from build123d import *

# Parameters (mm, degrees)
SKETCH1_R           = 47.5
BOSS_EXTRUDE1_DEPTH = 200
SKETCH2_R           = 30
CUT_EXTRUDE2_DEPTH  = 200
SKETCH4_R           = 47.5
BOSS_EXTRUDE2_DEPTH = 62.5
SKETCH5_R           = 5
CUT_EXTRUDE3_DEPTH  = 20
SKETCH6_R           = 27
CUT_EXTRUDE4_DEPTH  = 4


with BuildPart() as part:
    # Sketch1 → Boss-Extrude1 (new body)
    with BuildSketch(Plane(origin=(0, 0, 0), x_dir=(1, 0, 0), z_dir=(0, 1, 0))):
        with Locations(Location((0, 0, 0), (0, 0, 270))):
            Circle(SKETCH1_R)
    extrude(amount=BOSS_EXTRUDE1_DEPTH)

    # Sketch2 → Cut-Extrude2 (cut)
    with BuildSketch(Plane(origin=(0, 200, 0), x_dir=(1, 0, 0), z_dir=(0, 1, 0))):
        with Locations(Location((0, 0, 0), (0, 0, 270))):
            Circle(SKETCH2_R)
    extrude(amount=-CUT_EXTRUDE2_DEPTH, mode=Mode.SUBTRACT)

    # Sketch4 → Boss-Extrude2 (add)
    with BuildSketch(Plane.XY):
        with Locations((0, 100)):
            Circle(SKETCH4_R)
    extrude(amount=BOSS_EXTRUDE2_DEPTH)

    # Sketch5 → Cut-Extrude3 (cut)
    with BuildSketch(Plane.XY.offset(62.5)):
        with Locations((0, 138)):
            Circle(SKETCH5_R)
        with Locations((0, 62)):
            Circle(SKETCH5_R)
        with Locations((38, 100)):
            Circle(SKETCH5_R)
        with Locations((-38, 100)):
            Circle(SKETCH5_R)
    extrude(amount=-CUT_EXTRUDE3_DEPTH, mode=Mode.SUBTRACT)

    # Sketch6 → Cut-Extrude4 (cut)
    with BuildSketch(Plane.XY.offset(62.5)):
        with Locations((0, 100)):
            Circle(SKETCH6_R)
    extrude(amount=-CUT_EXTRUDE4_DEPTH, mode=Mode.SUBTRACT)


solid = part.part
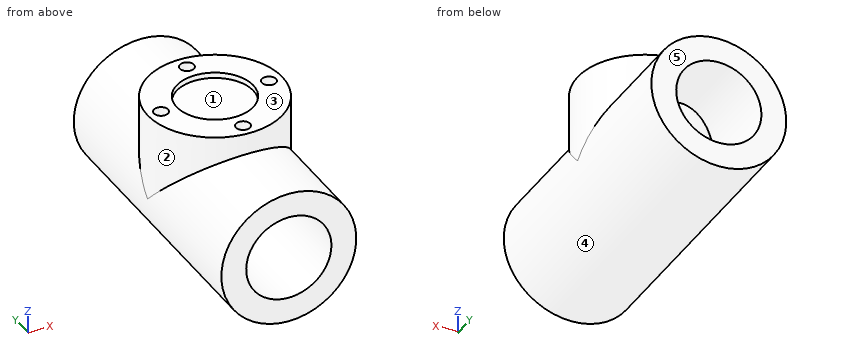
Source: CAD feature listing. Evaluate the final solid. Frame: model axes, mm. Face numbers are marked on the shaded views. A direction names the side the tool comes from. Give positions to 0.01 mm unless a question says otherwise; leave off trailing zeros. Loops run counter-clockwise (first coordinate to the right, second up) from the corner with the lowest first, then second, coordinate; pieces in that order, holes last. Notation, with made-up numbers: (51.25, 63.5) -> (74.25, 63.5) arc R22 ccw to (74.25, 82.5) -> close; hole circle Ø5 at (46, -30). An arc over 180 degrees is marked (long way). Use a Markdown table: item, result. Add a question column.
1) Reachability of the marked faces 4 and 5 from +Z, -Z, +X, -X, +Y, -Y: full face, straight path, thin tool, end or side. Return the list, or none.
2) First-contact query: pin 1 (12 mm diameter, centred on y = 60.5, z = -21, fed in from +X); pin 2 (5 mm diameter, centred on x = -37, y = 102, fed in from +Z); pin 3 (5 mm diameter, centred on y = 44.5, z = 45, fed in from -X). Flat tips, straight axial feed; report the tip coordinate or a pass-through.
3) Section query C-C, the plane x = -38. Return the cut outline in (y, z), then the cut area to 3 significant figures.
4) Pull-direction query (X, two-part tool) for the marked faces 1, 2 and 3; classes: +X half, -X half, draft (parallel to the pull), parting line (faces both ways), or undercut.
5) Section query D-D, the plane z = -23.5. Return the cut outline in (x, y), then the cut area to 3 significant figures.
6) Section query A-A, the plane x = 0. Return the cut outline in (y, z).
7) Line query: line 1 along Y through (x, z) = (0, 59); line 2 along Z through (x, y) = (-12, 88.5); line 3 along Z through (x, y) = (27.5, 104). Output: solid intervals per line, ascending. Write a range as [from, to].
8) Section query B-B, the plane y = 100. Return the cut outline in (x, z), then the cut area to 3 significant figures.
Numbers:
| question | item | result |
|---|---|---|
| 1 | face 4 | none |
| 1 | face 5 | +Z, -Z, +X, -X, +Y |
| 2 | pin 1 | stops at x = 45.07 |
| 2 | pin 2 | stops at z = 42.5 |
| 2 | pin 3 | stops at x = -21.21 |
| 3 | outline | (0, -28.5) -> (200, -28.5) -> (200, 28.5) -> (128.5, 28.5) -> (128.5, 62.5) -> (105, 62.5) -> (105, 42.5) -> (95, 42.5) -> (95, 62.5) -> (71.5, 62.5) -> (71.5, 28.5) -> (0, 28.5) -> close |
| 3 | area | 13,100 mm2 |
| 4 | face 1 | undercut |
| 4 | face 2 | parting line |
| 4 | face 3 | draft |
| 5 | outline | (-41.28, 0) -> (-18.65, 0) -> (-18.65, 200) -> (-41.28, 200) -> close; (18.65, 0) -> (41.28, 0) -> (41.28, 200) -> (18.65, 200) -> close |
| 5 | area | 9,050 mm2 |
| 6 | outline | (0, -47.5) -> (200, -47.5) -> (200, -30) -> (0, -30) -> close; (0, 30) -> (52.5, 30) -> (52.5, 0) -> (147.5, 0) -> (147.5, 30) -> (200, 30) -> (200, 47.5) -> (147.5, 47.5) -> (147.5, 62.5) -> (143, 62.5) -> (143, 42.5) -> (133, 42.5) -> (133, 62.5) -> (127, 62.5) -> (127, 58.5) -> (73, 58.5) -> (73, 62.5) -> (67, 62.5) -> (67, 42.5) -> (57, 42.5) -> (57, 62.5) -> (52.5, 62.5) -> (52.5, 47.5) -> (0, 47.5) -> close |
| 7 | line 1 | y = [52.5, 57], [67, 73], [127, 133], [143, 147.5] |
| 7 | line 2 | z = [-45.96, -27.5], [0, 58.5] |
| 7 | line 3 | z = [-38.73, -11.99], [0, 62.5] |
| 8 | outline | (-47.5, 0) arc R47.5 ccw to (47.5, 0) -> (47.5, 62.5) -> (43, 62.5) -> (43, 42.5) -> (33, 42.5) -> (33, 62.5) -> (27, 62.5) -> (27, 58.5) -> (-27, 58.5) -> (-27, 62.5) -> (-33, 62.5) -> (-33, 42.5) -> (-43, 42.5) -> (-43, 62.5) -> (-47.5, 62.5) -> close; hole (-30, 0) arc R30 ccw to (30, 0) -> close |
| 8 | area | 7,450 mm2 |
